Geometry: final body of the model. Coordinates: model frame, mm. Give positions to 0.01 mm unless a question says otherwise; leave off trailing zeros. Loops run counter-clockwise (first coordinate to the right, second up) from the corner with the lowest first, then second, coordinate; pieces in that order, holes last. Notation, with made-up numbers: (51, 12.5) - (62, 12.5) arc R23 cw to (62, 49.5) - close; hole circle Ø4 at (-37, 2.25). An arc over 180 degrees is marked (long way). Use one line per item in the form item = value.
Solid Edge part; units mm, degrees
sketch "Sketch1" plane through (0, 0, 0) normal (0, -1, 0) x (1, 0, 0)
  line L0 (35, 25) -> (-35, 25)
  line L1 (-35, 25) -> (-35, -25)
  line L2 (-35, -25) -> (35, -25)
  line L3 (35, -25) -> (35, 25)
extrude "Protrusion1" add sketch "Sketch1" along normal blind 10
sketch "Sketch2" plane through (0, 0, 0) normal (0, -1, 0) x (1, 0, 0)
  circle A0 centre (-17.5183, 0) radius 2.5
extrude "ExtrudedCutout_3" cut sketch "Sketch2" along normal blind 10
sketch "Sketch3" plane through (0, 0, 0) normal (0, -1, 0) x (1, 0, 0)
  circle A0 centre (17.5183, 0) radius 2.5
extrude "ExtrudedCutout_4" cut sketch "Sketch3" along normal blind 10
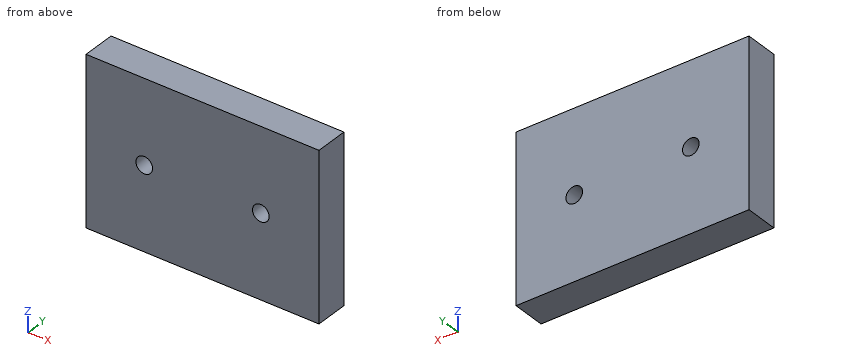
(1) Material intervals for L1, parallel to X at y = -9, z = -2; L2, parallel to Z at x = -17, y = -2, sorted ascending. Write a range as from..to.
Solution:
L1 = -35..-19.02, -16.02..16.02, 19.02..35
L2 = -25..-2.45, 2.45..25
(2) Cut plane A-A (z = 0). Return the cut outline in (x, y).
Solution:
outline = (-35, -10) - (-20.02, -10) - (-20.02, 0) - (-35, 0) - close; (-15.02, -10) - (15.02, -10) - (15.02, 0) - (-15.02, 0) - close; (20.02, -10) - (35, -10) - (35, 0) - (20.02, 0) - close
(3) Cut plane C-C (x = -17). Return the cut outline in (y, z).
Solution:
outline = (-10, -25) - (0, -25) - (0, -2.45) - (-10, -2.45) - close; (-10, 2.45) - (0, 2.45) - (0, 25) - (-10, 25) - close
(4) Cut plane B-B (x = 16.5). Return the cut outline in (y, z), plus the area to 3 significant figures.
Solution:
outline = (-10, -25) - (0, -25) - (0, -2.28) - (-10, -2.28) - close; (-10, 2.28) - (0, 2.28) - (0, 25) - (-10, 25) - close
area = 454 mm2
